```python
from build123d import *

# Parameters (mm, degrees)
SKETCH1_W           = 7
SKETCH1_H           = 7
BOSS_EXTRUDE1_DEPTH = 3
SKETCH3_W           = 10
SKETCH3_H           = 10
BOSS_EXTRUDE2_DEPTH = 15
BOSS_EXTRUDE4_DEPTH = 4


with BuildPart() as part:
    # Sketch1 → Boss-Extrude1 (new body)
    with BuildSketch(Plane(origin=(0, 0, 0), x_dir=(1, 0, 0), z_dir=(0, 1, 0))):
        Rectangle(SKETCH1_W, SKETCH1_H)
    extrude(amount=BOSS_EXTRUDE1_DEPTH)

    # Sketch3 → Boss-Extrude2 (add)
    with BuildSketch(Plane(origin=(0, 3, 0), x_dir=(1, 0, 0), z_dir=(0, 1, 0))):
        Rectangle(SKETCH3_W, SKETCH3_H)
    extrude(amount=BOSS_EXTRUDE2_DEPTH)

    # Sketch4 → Boss-Extrude4 (add)
    with BuildSketch(Plane(origin=(0, 18, 0), x_dir=(1, 0, 0), z_dir=(0, 1, 0))):
        Polygon((10.857439738, 43.294473551), (10.857439738, 53.294473551), (0.857439738, 53.294473551), (0.857439738, 43.294473551), (-35.642560262, 43.294473551), (-35.642560262, -43.294473551), (0.857439738, -43.294473551), (0.857439738, -53.294473551), (10.857439738, -53.294473551), (10.857439738, -43.294473551), (47.357439738, -43.294473551), (47.357439738, -5), (57.357439738, -5), (57.357439738, 5), (47.357439738, 5), (47.357439738, 43.294473551), align=None)
    extrude(amount=BOSS_EXTRUDE4_DEPTH)


solid = part.part
```
Check sheet for the modelled part. Datum: model origin and axes. Units: mm. A direction names the side the tool comes from. Round coordinates to 2 decimals unless told otherwise and drop trailing zeros. Order: outer loops, then holes, each group sorted by start corner. A loop starts at its lowest first (then second) coordinate and runs counter-clockwise, first axis right, second up.
1) Tool access check on faces 1 (the flat face through (10.857, 20, 48)), 2 (the flat face through (29, 20, -43.294)), 3 (the flat face through (0, 10, 5)), 4 (the flat face through (-18, 20, 43.294)). Record the directions out of +Z, -Z, +X, -X, +Y, -Y that give a thin tool (end or side, any length) a straight path to the whole face; none if there is none.
2) Section check C-C (z = -29.5). Record the boundary of the cut face in (x, y), and give its area (3 significant figures).
3) Go/stop test with flat-tipped pins: pin 1 Ø1 at (x, y) = (-0.5, 16.5) entering from -Z; pin 2 Ø0.9 at (y, z) = (1.5, 1.5) entering from +X; pin 3 Ø1.2 at (y, z) = (19.5, -46.5) entering from +X. Record where each tip stops, or that it passes through.
4) Section check B-B (x = -0.5). Record the boundary of the cut face in (y, z).
5) Scan lines: line 1 (X direction, y = 15.5, z = -1); line 2 (Z direction, x = 37, y = 20.5); line 3 (Y direction, x = 36, z = 28). Record each from-to range of solid material in increasing order.
6) Section check D-D (x = 50). Record the boundary of the cut face in (y, z).
7) Section check A-A (y = 20.25). Record the boundary of the cut face in (x, z).
Result:
1. face 1: +Z, +X, +Y, -Y
1. face 2: -Z, +X, +Y, -Y
1. face 3: +Z, +X, -X, -Y
1. face 4: +Z, -X, +Y, -Y
2. outline: (-35.64, 18) - (47.36, 18) - (47.36, 22) - (-35.64, 22) - close
2. area: 332 mm2
3. pin 1: stops at z = -5
3. pin 2: stops at x = 3.5
3. pin 3: stops at x = 10.86
4. outline: (0, -3.5) - (3, -3.5) - (3, -5) - (18, -5) - (18, -43.29) - (22, -43.29) - (22, 43.29) - (18, 43.29) - (18, 5) - (3, 5) - (3, 3.5) - (0, 3.5) - close
5. line 1: x = -5 to 5
5. line 2: z = -43.29 to 43.29
5. line 3: y = 18 to 22
6. outline: (18, -5) - (22, -5) - (22, 5) - (18, 5) - close
7. outline: (-35.64, -43.29) - (0.86, -43.29) - (0.86, -53.29) - (10.86, -53.29) - (10.86, -43.29) - (47.36, -43.29) - (47.36, -5) - (57.36, -5) - (57.36, 5) - (47.36, 5) - (47.36, 43.29) - (10.86, 43.29) - (10.86, 53.29) - (0.86, 53.29) - (0.86, 43.29) - (-35.64, 43.29) - close
